The figure shows three views and two pictorial views of one solid part (mm, origin at its lowest corner). Answer the questions. A direction names the side the tool comes from. Round coordinates to 2 decimals unless told otherwise and drop trailing zeros. Write each loop counter-clockwise with the first axis right and the second up, starting at its lowest first coordinate (ties: lowest second). Pieces come first, ordered by that corner, then holes.
Item 1: For a pull along X with two mould halves and no side action, classify the marked faces 3 and 4 as +X half, -X half, draft (parallel to the pull), parting line (faces both ways), or undercut.
Item 2: Find section C-C on y = 17.5. Give the vertices of the cut face in (x, z), then the cut area to 3 significant figures.
Item 3: Find section A-A on z = 3.5. Give the vertices of the cut face in (x, y).
Item 4: Find the intervals of material crossed by probe 1 along Z at (x, y) = (17.5, 14.5); probe 2 along Y at (x, z) = (20.5, 0.75); probe 3 along Y at (x, z) = (8.5, 5.5), in increasing order.
Item 5: A tool of negligible diameter and unlimited length cuts with its end or side. For the marked faces 1 and 2, from which of +Z, -Z, +X, -X, +Y, -Y can it reach the whole face along a straight path? Write none if from no direction.
Item 6: Find section B-B on x = 10. Give the vertices of the cut face in (y, z).
Item 7: Find section D-D on x = 37. Give the vertices of the cut face in (y, z), then the cut area to 3 significant figures.
Item 8: Each of these flat-tipped pins is pushed along its axis until it touches: pin 1 (5 mm diameter, centred on x = 34.5, y = 17.5, fed in from +Z); pin 2 (3 mm diameter, centred on x = 11.5, z = 4, fed in from -Y). Where does it stop, or does it pass through?
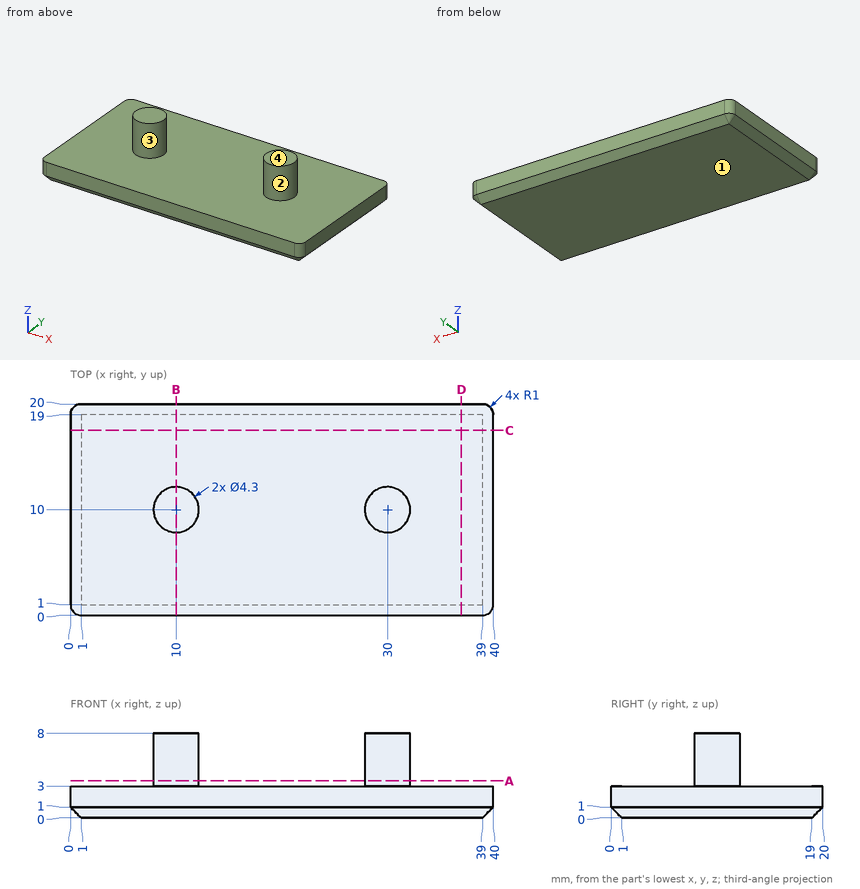
Check values:
1. face 3: undercut
1. face 4: draft
2. outline: (0, 1) - (1, 0) - (39, 0) - (40, 1) - (40, 3) - (0, 3) - close
2. area: 119 mm2
3. outline: circle Ø4.3 at (10, 10); circle Ø4.3 at (30, 10)
4. probe 1: z = 0 to 3
4. probe 2: y = 0.25 to 19.75
4. probe 3: y = 8.46 to 11.54
5. face 1: -Z, +X, -X, +Y, -Y
5. face 2: +Z
6. outline: (0, 1) - (1, 0) - (19, 0) - (20, 1) - (20, 3) - (12.15, 3) - (12.15, 8) - (7.85, 8) - (7.85, 3) - (0, 3) - close
7. outline: (0, 1) - (1, 0) - (19, 0) - (20, 1) - (20, 3) - (0, 3) - close
7. area: 59.0 mm2
8. pin 1: stops at z = 3
8. pin 2: stops at y = 0
